Verification items for the finished model (mm, model axes). Coordinates: 2 decimals unless noted, no trailing zeros. Write each loop counter-clockwise with the first axis right and the second up, starting at its lowest first coordinate (ties: lowest second). Pieces come first, ordered by that corner, then holes. Notation, with made-up numbers: (67.5, 15) -> (85.5, 15) arc R17 ccw to (85.5, 35) -> close; hole circle Ø4 at (88, -28.5). An arc over 180 degrees is marked (long way). Use CSV: the item, a comma, the result in double quotes.
```python
from build123d import *

# Parameters (mm, degrees)
SKETCH1_R           = 4
SKETCH1_R_2         = 2.5
BOSS_EXTRUDE1_DEPTH = 5


with BuildPart() as part:
    # Sketch1 → Boss-Extrude1 (new body)
    with BuildSketch(Plane.XY):
        Polygon((0, 0), (39, 0), (81, 0), (120, 0), (120, -70), (0, -70), align=None)
        with Locations((35, -55)):
            Circle(SKETCH1_R, mode=Mode.SUBTRACT)
        with Locations(Location((85, -55, 0), (0, 0, 180))):
            Circle(SKETCH1_R, mode=Mode.SUBTRACT)
        with Locations((10, -10)):
            Circle(SKETCH1_R_2, mode=Mode.SUBTRACT)
        with Locations(Location((110, -10, 0), (0, 0, 180))):
            Circle(SKETCH1_R_2, mode=Mode.SUBTRACT)
        with Locations((110, -60)):
            Circle(SKETCH1_R_2, mode=Mode.SUBTRACT)
        with Locations(Location((10, -60, 0), (0, 0, 180))):
            Circle(SKETCH1_R_2, mode=Mode.SUBTRACT)
        with Locations((30, -14.5)):
            Circle(SKETCH1_R_2, mode=Mode.SUBTRACT)
        with Locations(Location((90, -14.5, 0), (0, 0, 180))):
            Circle(SKETCH1_R_2, mode=Mode.SUBTRACT)
    extrude(amount=BOSS_EXTRUDE1_DEPTH)


solid = part.part
```
1) Mould release check, pull along Y, two halves, no side actions. Record for faces 1 (the flat face through (61, -35, 0)), 2 (the flat face through (61, -70, 2)), 3 (the cylindrical face through (112.385, -59.249, 2.465)): released by +Y, released by -Y, zero draft, split by the parting line, or undercut.
Return value:
face 1,"zero draft"
face 2,"released by -Y"
face 3,"undercut"
2) Cross-section at B-B (x = 110). Record the boundary of the cut face in (y, z).
Return value:
outline,"(-70, 0) -> (-62.5, 0) -> (-62.5, 5) -> (-70, 5) -> close; (-57.5, 0) -> (-12.5, 0) -> (-12.5, 5) -> (-57.5, 5) -> close; (-7.5, 0) -> (0, 0) -> (0, 5) -> (-7.5, 5) -> close"
3) Cross-section at A-A (y = -10). Record the boundary of the cut face in (x, z), plus the area to 3 significant figures.
Return value:
outline,"(0, 0) -> (7.5, 0) -> (7.5, 5) -> (0, 5) -> close; (12.5, 0) -> (107.5, 0) -> (107.5, 5) -> (12.5, 5) -> close; (112.5, 0) -> (120, 0) -> (120, 5) -> (112.5, 5) -> close"
area,"550 mm2"
4) Scan lines: L1, parallel to Y at x = 10, z = 3; L2, parallel to Y at x = 30, z = 2.2; L3, parallel to Y at x = 9, z = 2.75. Record each from-to range of solid material in increasing order.
Return value:
L1,"-70 to -62.5, -57.5 to -12.5, -7.5 to 0"
L2,"-70 to -17, -12 to 0"
L3,"-70 to -62.29, -57.71 to -12.29, -7.71 to 0"
5) Cross-section at C-C (z = 2.65). Give the number of separate pieces and of enclosed holes in the cut face, plus the area to 3 significant figures.
Return value:
separate pieces,"1"
enclosed holes,"8"
area,"8,180 mm2"
6) Cross-section at D-D (x = 85). Record the boundary of the cut face in (y, z).
Return value:
outline,"(-70, 0) -> (-59, 0) -> (-59, 5) -> (-70, 5) -> close; (-51, 0) -> (0, 0) -> (0, 5) -> (-51, 5) -> close"
7) Gauge pin test, flat end, axial feed: pin 1 (4 mm diameter, centred on x = 110, y = -10, fed in from -Z). Record the tip position at first contact, or that the pin passes through.
Return value:
pin 1,"through"
